For this review, take the finished solid that the model builds, in its own axes (mm). A direction names the side the tool comes from. Round coordinates to 2 decimals unless told otherwise and drop trailing zeros. Loops run counter-clockwise (first coordinate to the right, second up) from the corner with the lowest first, then second, coordinate; pieces in that order, holes last. Notation, with made-up numbers: (36, 85) -> (41, 85) arc R19 cw to (41, 107) -> close; hole circle Ø8 at (58.25, 19.25). An arc over 180 degrees is marked (long way). One line per question, with ' | ' between items. Start each with the question number.
1. Draft analysis for pull direction Y (two halves, no side actions). For faces 3 (the face through (13.51, -3.15, -2.41)), 4 (the face through (-2.958, 6.896, -4.056)), 5 (the face through (24.931, 0, 0)), state which applies: pulls with the +Y half, pulls with the -Y half, needs draft (parallel to the pull), parting line crosses it, or undercut.
2. Wall thickness on line 1 along X through (y, z) = (0.5, -0.25); line 2 along X through (y, z) = (8, -0.5); line 3 along X through (y, z) = (-1.5, 6.5): over which ranges is each line inside the solid? List them lowest first.
3. Consider section B-B (x = -0.5). Write out the cut boundary in (y, z), and give its area (3 significant figures).
4. For pin 1 Ø1 at (y, z) = (2, 5) entering from +X; pin 2 Ø6 at (x, z) = (3.5, -1) entering from +Y; pin 3 Ø10 at (x, y) = (5, 7.5) entering from +Z, all flat-tipped, find the tip position at first contact; note any pin that passes through.
5. Consider section C-C (x = 21). Write out the cut boundary in (y, z), and give its area (3 significant figures).
6. Consider section A-A (y = 0). Write out the cut boundary in (x, z), and give its area (3 significant figures).
7. For faces 1 (the face through (-6, 0, 0)), 2 (the face through (16.717, -1.5, 4.4)), list the 3-axis set-ups (+Z, -Z, +X, -X, +Y, -Y) from which the entire face can be reached by the end or side of a thin tool; tool diameter is ignored.
Autodesk Inventor part; units mm, degrees
ref_plane "YZ Plane" through (0, 0, 0) normal (1, 0, 0) x (0, 1, 0)
ref_plane "XZ Plane" through (0, 0, 0) normal (0, 1, 0) x (-1, 0, 0)
ref_plane "XY Plane" through (0, 0, 0) normal (0, 0, 1) x (1, 0, 0)
sketch "Sketch1" plane through (0, 0, 0) normal (0, 0, 1) x (1, 0, 0)
  line L0 (0, 0) -> (26.387, 0)
  line L1 (0, 0) -> (0, 4.969)
  line L2 (0, 4.969) -> (10.717, 4.969)
  line L3 (10.717, 4.969) -> (10.717, 3.968)
  line L4 (10.717, 3.968) -> (16.717, 3.968)
  line L5 (16.717, 3.968) -> (16.717, 7.2744)
  line L6 (16.717, 7.2744) -> (26.387, 2.558)
  line L7 (26.387, 2.558) -> (24.9308, 1.5)
  line L8 (24.9308, 1.5) -> (24.9308, 0)
  dimension "d0" = 10.717
  dimension "d1" = 9.938
  dimension "d2" = 7.936
  dimension "d3" = 6
  dimension "d4" = 5.116
  dimension "d6" = 26
  dimension "d8" = 9.67
  dimension "d9" = 36
  dimension "d10" = 3
revolve "Revolution1" add sketch "Sketch1" angle 360 about axis through (0, 0, 0) along (1, 0, 0)
sketch "Sketch2" plane through (0, 0, 0) normal (-1, 0, 0) x (0, 0, 1)
  circle A0 centre (0, 0) radius 4.969
  line L0 (0, 9.2376) -> (8, 4.6188)
  line L1 (8, 4.6188) -> (8, -4.6188)
  line L2 (8, -4.6188) -> (0, -9.2376)
  line L3 (0, -9.2376) -> (-8, -4.6188)
  line L4 (-8, -4.6188) -> (-8, 4.6188)
  line L5 (-8, 4.6188) -> (0, 9.2376)
  dimension "d11" = 16
extrude "Extrusion1" add sketch "Sketch2" along normal blind 6 contours A0 | L0 L1 L2 L3 L4 L5
fillet "Fillet1" radius 0.5 2 edges at (16.717, -3.968, 0) (16.717, -7.2744, 0)
properties part number "212-05" material "Titanium"
Answer block:
1) face 3: parting line crosses it | face 4: pulls with the +Y half | face 5: undercut
2) line 1: x = -6 to 24.93 | line 2: x = -6 to 0 | line 3: x = -6 to 0, 16.76 to 17.95
3) outline: (-9.24, 0) -> (-4.62, -8) -> (4.62, -8) -> (9.24, 0) -> (4.62, 8) -> (-4.62, 8) -> close | area: 222 mm2
4) pin 1: stops at x = 21.62 | pin 2: stops at y = 4.97 | pin 3: stops at z = 4.29
5) outline: circle Ø10.37 at (0, 0) | area: 84.5 mm2
6) outline: (-6, -8) -> (0, -8) -> (0, -4.97) -> (10.72, -4.97) -> (10.72, -3.97) -> (16.22, -3.97) arc R0.5 cw to (16.72, -4.47) -> (16.72, -6.47) arc R0.5 ccw to (17.44, -6.92) -> (26.39, -2.56) -> (24.93, -1.5) -> (24.93, 1.5) -> (26.39, 2.56) -> (17.44, 6.92) arc R0.5 ccw to (16.72, 6.47) -> (16.72, 4.47) arc R0.5 cw to (16.22, 3.97) -> (10.72, 3.97) -> (10.72, 4.97) -> (0, 4.97) -> (0, 8) -> (-6, 8) -> close | area: 339 mm2
7) face 1: +Z, -Z, -X, +Y, -Y | face 2: none
